Here's how the part is built. I have some questions about the finished solid (model axes, mm). Face numbers are marked on the shaded views. Coordinates: 2 decimals unless noted, no trailing zeros.
Item 1: We'd pull the mould along Z, two halves only. Please class the marked faces 1, 2 and 3: +Z half, -Z half, draft (parallel to the pull), parting line (faces both ways), or undercut.
Item 2: If I drill on line 1 (X direction, y = 0.25, z = 0); line 2 (X direction, y = 0.9, z = 0); line 3 (Y direction, x = -12, z = -34), over which ranges is the centre line in solid material (lowest first)?
Item 3: I'm going to push flat-ended pins straight in: pin 1 Ø1 at (x, y) = (-11.5, 2.5) entering from -Z; pin 2 Ø10 at (x, z) = (-26, 7.5) entering from +Y; pin 3 Ø1.5 at (x, y) = (-41, 4) entering from -Z. Where does each tip first touch, or does it pass through?
Item 4: If we section it at A-A (y = 4.25): Count the separate pieces of the cut face and the enclosed holes in it, then the cut area to 3 significant figures.
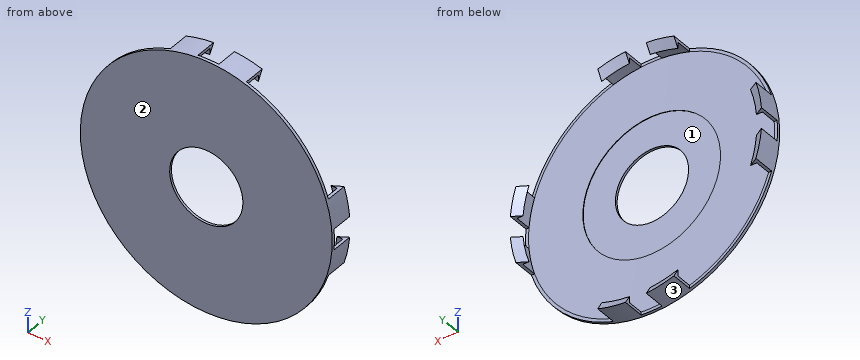
from build123d import *
from build123d.topology import SkipClean

# Parameters (mm, degrees)
CUT_EXTRUDE_1_REACH = 63.375
SKETCH_3_W          = 7.1
SKETCH_3_H          = 24.266407169
SKETCH_3_W_2        = 24.266407169
SKETCH_3_H_2        = 7.1
SKETCH_4_R          = 23.5
CUT_EXTRUDE_2_DEPTH = 7.5


with BuildPart() as part:
    # Эскиз2 → Повернуть1 (revolve)
    with BuildSketch(Plane.XY, mode=Mode.PRIVATE) as revolve_1_sk:
        Polygon((12.5, 0), (12.5, 0.896852554), (42, 1), (42, 6.5), (40, 6.5), (43, 8.3), (43, 0), align=None)
    revolve(revolve_1_sk.sketch.rotate(Axis((0, -20.602437041, 0), (0, 1, 0)), 90), axis=Axis((0, -20.602437041, 0), (0, 1, 0)))

    # Вырез-Вытянуть1: up to this cone (the profile starts inside it)
    with SkipClean():  # the faces are left unmerged after this step: merging them gives an invalid solid
        cut_extrude_1_end = Plane(origin=(0, 8.3, 0), z_dir=(0, 1, 0)).offset(-7.446852991) * Cone(0.000285998, 629513.797627356, 2201.109848989, align=(Align.CENTER, Align.CENTER, Align.MIN), mode=Mode.PRIVATE)
        # Эскиз3 → Вырез-Вытянуть1 (cut, up to the surface)
        with BuildSketch(Plane(origin=(0, 8.3, 0), x_dir=(1, 0, 0), z_dir=(0, 1, 0)), mode=Mode.PRIVATE) as cut_extrude_1_sk1:
            Polygon((-13, -13), (-53, -13), (-13, -53), align=None)
        cut_extrude_1_tool1 = extrude(cut_extrude_1_sk1.sketch, amount=-CUT_EXTRUDE_1_REACH, mode=Mode.PRIVATE) & cut_extrude_1_end
        add(cut_extrude_1_tool1.solids().sort_by_distance((-26.333333, 8.3, 26.333333))[0], mode=Mode.SUBTRACT)
        # Эскиз3 → Вырез-Вытянуть1 (cut, up to the surface)
        with BuildSketch(Plane(origin=(0, 8.3, 0), x_dir=(1, 0, 0), z_dir=(0, 1, 0)), mode=Mode.PRIVATE) as cut_extrude_1_sk2:
            Polygon((-13, 13), (-13, 53), (-53, 13), align=None)
        cut_extrude_1_tool2 = extrude(cut_extrude_1_sk2.sketch, amount=-CUT_EXTRUDE_1_REACH, mode=Mode.PRIVATE) & cut_extrude_1_end
        add(cut_extrude_1_tool2.solids().sort_by_distance((-26.333333, 8.3, -26.333333))[0], mode=Mode.SUBTRACT)
        # Эскиз3 → Вырез-Вытянуть1 (cut, up to the surface)
        with BuildSketch(Plane(origin=(0, 8.3, 0), x_dir=(1, 0, 0), z_dir=(0, 1, 0)), mode=Mode.PRIVATE) as cut_extrude_1_sk3:
            Polygon((13, 13), (53, 13), (13, 53), align=None)
        cut_extrude_1_tool3 = extrude(cut_extrude_1_sk3.sketch, amount=-CUT_EXTRUDE_1_REACH, mode=Mode.PRIVATE) & cut_extrude_1_end
        add(cut_extrude_1_tool3.solids().sort_by_distance((26.333333, 8.3, -26.333333))[0], mode=Mode.SUBTRACT)
        # Эскиз3 → Вырез-Вытянуть1 (cut, up to the surface)
        with BuildSketch(Plane(origin=(0, 8.3, 0), x_dir=(1, 0, 0), z_dir=(0, 1, 0)), mode=Mode.PRIVATE) as cut_extrude_1_sk4:
            Polygon((13, -13), (13, -53), (53, -13), align=None)
        cut_extrude_1_tool4 = extrude(cut_extrude_1_sk4.sketch, amount=-CUT_EXTRUDE_1_REACH, mode=Mode.PRIVATE) & cut_extrude_1_end
        add(cut_extrude_1_tool4.solids().sort_by_distance((26.333333, 8.3, 26.333333))[0], mode=Mode.SUBTRACT)
        # Эскиз3 → Вырез-Вытянуть1 (cut, up to the surface)
        with BuildSketch(Plane(origin=(0, 8.3, 0), x_dir=(1, 0, 0), z_dir=(0, 1, 0)), mode=Mode.PRIVATE) as cut_extrude_1_sk5:
            with Locations((0, 40.866796416)):
                Rectangle(SKETCH_3_W, SKETCH_3_H)
        cut_extrude_1_tool5 = extrude(cut_extrude_1_sk5.sketch, amount=-CUT_EXTRUDE_1_REACH, mode=Mode.PRIVATE) & cut_extrude_1_end
        add(cut_extrude_1_tool5.solids().sort_by_distance((0, 8.3, -40.866796))[0], mode=Mode.SUBTRACT)
        # Эскиз3 → Вырез-Вытянуть1 (cut, up to the surface)
        with BuildSketch(Plane(origin=(0, 8.3, 0), x_dir=(1, 0, 0), z_dir=(0, 1, 0)), mode=Mode.PRIVATE) as cut_extrude_1_sk6:
            with Locations((-40.866796416, 0)):
                Rectangle(SKETCH_3_W_2, SKETCH_3_H_2)
        cut_extrude_1_tool6 = extrude(cut_extrude_1_sk6.sketch, amount=-CUT_EXTRUDE_1_REACH, mode=Mode.PRIVATE) & cut_extrude_1_end
        add(cut_extrude_1_tool6.solids().sort_by_distance((-40.866796, 8.3, 0))[0], mode=Mode.SUBTRACT)
        # Эскиз3 → Вырез-Вытянуть1 (cut, up to the surface)
        with BuildSketch(Plane(origin=(0, 8.3, 0), x_dir=(1, 0, 0), z_dir=(0, 1, 0)), mode=Mode.PRIVATE) as cut_extrude_1_sk7:
            with Locations((40.866796416, 0)):
                Rectangle(SKETCH_3_W_2, SKETCH_3_H_2)
        cut_extrude_1_tool7 = extrude(cut_extrude_1_sk7.sketch, amount=-CUT_EXTRUDE_1_REACH, mode=Mode.PRIVATE) & cut_extrude_1_end
        add(cut_extrude_1_tool7.solids().sort_by_distance((40.866796, 8.3, 0))[0], mode=Mode.SUBTRACT)
        # Эскиз3 → Вырез-Вытянуть1 (cut, up to the surface)
        with BuildSketch(Plane(origin=(0, 8.3, 0), x_dir=(1, 0, 0), z_dir=(0, 1, 0)), mode=Mode.PRIVATE) as cut_extrude_1_sk8:
            with Locations((0, -40.866796416)):
                Rectangle(SKETCH_3_W, SKETCH_3_H)
        cut_extrude_1_tool8 = extrude(cut_extrude_1_sk8.sketch, amount=-CUT_EXTRUDE_1_REACH, mode=Mode.PRIVATE) & cut_extrude_1_end
        add(cut_extrude_1_tool8.solids().sort_by_distance((0, 8.3, 40.866796))[0], mode=Mode.SUBTRACT)

    # Эскиз4 → Вырез-Вытянуть2 (cut)
    with SkipClean():  # the faces are left unmerged after this step: merging them gives an invalid solid
        with BuildSketch(Plane(origin=(0, 8.3, 0), x_dir=(1, 0, 0), z_dir=(0, 1, 0))):
            with Locations(Location((0, 0, 0), (0, 0, 270))):
                Circle(SKETCH_4_R)
        extrude(amount=-CUT_EXTRUDE_2_DEPTH, mode=Mode.SUBTRACT)


solid = part.part
Answer list:
1. face 1: undercut
1. face 2: draft
1. face 3: parting line
2. line 1: x = -43 to -12.5, 12.5 to 43
2. line 2: x = -43 to -23.5, 23.5 to 43
2. line 3: y = 0 to 0.98
3. pin 1: stops at z = -41.57
3. pin 2: stops at y = 0.97
3. pin 3: stops at z = -13
4. separate pieces: 8
4. enclosed holes: 0
4. area: 77.3 mm2
